The model under review builds one solid part; all positions refer to its coordinate system, in mm. A direction names the side the tool comes from. Coordinates: 2 decimals unless noted, no trailing zeros. Loops run counter-clockwise (first coordinate to the right, second up) from the corner with the lowest first, then second, coordinate; pieces in that order, holes last. Notation, with made-up numbers: (24, -23) - (52, -23) arc R11 cw to (52, -2) - close; hole circle Ø5 at (67, 72). An arc over 180 degrees is marked (long way). One line per item, written item: value. Start each with the question number.
1. We need section A-A, the plane y = 2.54. Give the boundary of the cut face in (x, z).
2. We need section D-D, the plane x = 14. Give the boundary of the cut face in (y, z).
3. We need section C-C, the plane y = -9. Give the boundary of the cut face in (x, z), then the cut area to 3 significant figures.
4. To check wall thickness, follow line 1 (Z direction, x = 0.5, y = 1); line 2 (X direction, y = -16.5, z = 6.5); line 3 (Y direction, x = 20.5, z = 5). State the ranges of each line that lie inside material, in increasing order.
5. We need section B-B, the plane z = 0. Give the boundary of the cut face in (x, y).
6. For faces 1 (the face through (35.56, -16, 0)), 2 (the face through (0, -5.08, 0)), 3 (the face through (0, 4, -6.693)), list the 3-axis set-ups (+Z, -Z, +X, -X, +Y, -Y) from which the entire face can be reached by the end or side of a thin tool; tool diameter is ignored.
7. Insertion check: P1, Ø6, axis at x = -24.5, z = 4.5, coming from the +Y side; P2, Ø3, axis at x = -3.5, z = -1.5, coming from the -Y side; P3, Ø6, axis at y = 1, z = -3.5, coming from the -X side. Each pin has a flat end and moves straight along its axis. Give the tip position at first contact, or say it passes through.
8. Mouldability with a two-part tool opening along X and no side actions: class faces 4 (the face through (-27.94, -18, 0)), 5 (the face through (31.803, -31.747, 0.251)), 6 (the face through (-35.56, -16, 0)) as +X half, -X half, draft (parallel to the pull), parting line (faces both ways), or undercut.
from build123d import *

# Parameters (mm, degrees)
F0_W      = 71.12
F0_H      = 22.86
F1_DEPTH  = 5.08
F2_W      = 7.62
F2_H      = 22.86
F3_DEPTH  = 15.24
F4_R      = 11.43
F5_DEPTH  = 7.62
F6_R      = 11.43
F7_DEPTH  = 7.62
F8_R      = 7.62
F9_DEPTH  = 4.7371
F10_R     = 7.62
F11_DEPTH = 4.7371


with BuildPart() as f1:
    # F0 (on Front) → F1 (new body)
    with BuildSketch(Plane.XZ):
        Rectangle(F0_W, F0_H)
    extrude(amount=F1_DEPTH)

    # F2 (on face) → F3 (join)
    with BuildSketch(Plane.XZ.offset(5.08)):
        with Locations((-31.75, 0)):
            Rectangle(F2_W, F2_H)
        with Locations((31.75, 0)):
            Rectangle(F2_W, F2_H)
    extrude(amount=F3_DEPTH)

    # F4 (on face) → F5 (join)
    with BuildSketch(Plane.YZ.offset(35.56)):
        with Locations((-20.32, 0)):
            Circle(F4_R)
    extrude(amount=-F5_DEPTH)

    # F6 (on face) → F7 (join)
    with BuildSketch(Plane(origin=(-35.56, 0, 0), x_dir=(0, -1, 0), z_dir=(-1, 0, 0))):
        with Locations((20.32, 0)):
            Circle(F6_R)
    extrude(amount=-F7_DEPTH)

    # F8 (on face) → F9 (join)
    with BuildSketch(Plane.XY.offset(11.43)):
        with Locations((0, 2.54)):
            Circle(F8_R)
    extrude(amount=-F9_DEPTH)

    # F10 (on face) → F11 (join)
    with BuildSketch(Plane(origin=(0, 0, -11.43), x_dir=(1, 0, 0), z_dir=(0, 0, -1))):
        with Locations((0, -2.54)):
            Circle(F10_R)
    extrude(amount=-F11_DEPTH)


solid = f1.part
Findings below:
1. outline: (-7.62, -11.43) - (7.62, -11.43) - (7.62, -6.69) - (-7.62, -6.69) - close; (-7.62, 6.69) - (7.62, 6.69) - (7.62, 11.43) - (-7.62, 11.43) - close
2. outline: (-5.08, -11.43) - (0, -11.43) - (0, 11.43) - (-5.08, 11.43) - close
3. outline: (-35.56, -11.43) - (-27.94, -11.43) - (-27.94, 11.43) - (-35.56, 11.43) - close; (27.94, -11.43) - (35.56, -11.43) - (35.56, 11.43) - (27.94, 11.43) - close
3. area: 348 mm2
4. line 1: -11.43 to -6.69, 6.69 to 11.43
4. line 2: -35.56 to -27.94, 27.94 to 35.56
4. line 3: -5.08 to 0
5. outline: (-35.56, -31.75) - (-27.94, -31.75) - (-27.94, -5.08) - (27.94, -5.08) - (27.94, -31.75) - (35.56, -31.75) - (35.56, 0) - (-35.56, 0) - close
6. face 1: +Z, -Z, +X, +Y, -Y
6. face 2: +Z, -Z, -Y
6. face 3: +X, -X, +Y
7. P1: y = 0
7. P2: y = -5.08
7. P3: x = -35.56
8. face 4: undercut
8. face 5: draft
8. face 6: -X half
